Job drawing, mm, ordinate dimensions from the low corner. One solid piece. A direction names the side the tool comes from. Coordinates: 2 decimals unless noted, no trailing zeros. Order: outer loops, then holes, each group sorted by start corner. A loop starts at its lowest first (then second) coordinate and runs counter-clockwise, first axis right, second up. Notation, with made-up numbers: (-5.5, 34.5) - (50.5, 34.5) arc R21 ccw to (50.5, 59.5) - close; hole circle Ø11 at (11.5, 65.5). An arc over 180 degrees is marked (long way). Return JSON: item names as keys, results as strings.
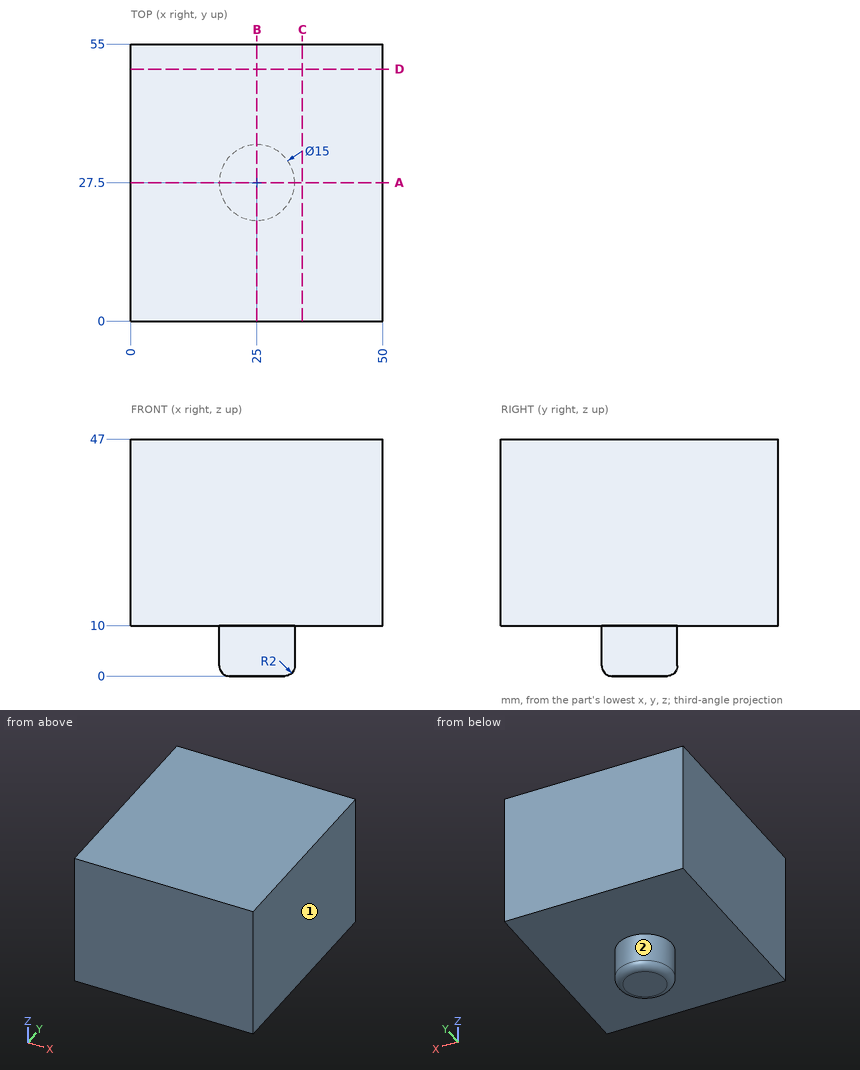
1. Probe L1, parallel to Z at x = 36.5, y = 17. List the from-to ranges inside material, lowest first.
Check values:
{"L1": "10 to 47"}
2. Cut at A-A on y = 27.5. Give the cut face in (x, z), plus the area to 3 significant figures.
Check values:
{"outline": "(0, 10) - (17.5, 10) - (17.5, 2) arc R2 ccw to (19.5, 0) - (30.5, 0) arc R2 ccw to (32.5, 2) - (32.5, 10) - (50, 10) - (50, 47) - (0, 47) - close", "area": "2,000 mm²"}
3. Cut at D-D on y = 50. Give the cut face in (x, z), plus the area to 3 significant figures.
Check values:
{"outline": "(0, 10) - (50, 10) - (50, 47) - (0, 47) - close", "area": "1,850 mm²"}
4. Cut at B-B on x = 25. Give the cut face in (y, z), plus the area to 3 significant figures.
Check values:
{"outline": "(0, 10) - (20, 10) - (20, 2) arc R2 ccw to (22, 0) - (33, 0) arc R2 ccw to (35, 2) - (35, 10) - (55, 10) - (55, 47) - (0, 47) - close", "area": "2,180 mm²"}
5. Cut at C-C on x = 34. Give the cut face in (y, z).
Check values:
{"outline": "(0, 10) - (55, 10) - (55, 47) - (0, 47) - close"}
6. Tool access for the marked faces 1 and 2: list every direction of +Z, -Z, +X, -X, +Y, -Y with a clear straight run to the whole face (end or side of a thin tool).
Check values:
{"face 1": "+Z, -Z, +X, +Y, -Y", "face 2": "-Z"}
